```python
from build123d import *

# Parameters (mm, degrees)
CROQUIS1_W                 = 35
CROQUIS1_H                 = 35
CROQUIS1_R                 = 1.25
SALIENTE_EXTRUIR1_DEPTH    = 5
SALIENTE_EXTRUIR2_DEPTH    = 35
CORTAR_EXTRUIR2_DEPTH      = 41.51542916
CORTAR_EXTRUIR2_DEPTH_BACK = 41.51542916
CROQUIS4_R                 = 1.25
CORTAR_EXTRUIR3_DEPTH      = 10
CROQUIS5_R                 = 3
CORTAR_EXTRUIR6_DEPTH      = 4.1


with BuildPart() as part:
    # Croquis1 → Saliente-Extruir1 (new body)
    with BuildSketch(Plane.XY):
        Rectangle(CROQUIS1_W, CROQUIS1_H)
        with Locations((15.37, -15.37)):
            Circle(CROQUIS1_R, mode=Mode.SUBTRACT)
        with Locations((-15.37, -15.37)):
            Circle(CROQUIS1_R, mode=Mode.SUBTRACT)
        with Locations((-15.37, 15.37)):
            Circle(CROQUIS1_R, mode=Mode.SUBTRACT)
        with Locations((15.37, 15.37)):
            Circle(CROQUIS1_R, mode=Mode.SUBTRACT)
    extrude(amount=SALIENTE_EXTRUIR1_DEPTH)

    # Croquis2 → Saliente-Extruir2 (add, through all)
    with BuildSketch(Plane(origin=(0, 17.5, 0), x_dir=(1, 0, 0), z_dir=(0, 1, 0))):
        with BuildLine():
            Line((17.5, -5), (17.5, -10.5))
            ThreePointArc((17.5, -10.5), (13.206356105, -6.465716172), (7.5, -5))
            Line((7.5, -5), (17.5, -5))
        make_face()
    extrude(amount=-SALIENTE_EXTRUIR2_DEPTH)

    # Croquis3 → Cortar-Extruir2 (cut, two sides: drawn at the far end of the back side and taken through both)
    with BuildSketch(Plane(origin=(0, 17.5, 0), x_dir=(1, 0, 0), z_dir=(0, 1, 0)).offset(-CORTAR_EXTRUIR2_DEPTH_BACK)):
        with BuildLine():
            Line((17.5, 0), (7.5, 0))
            ThreePointArc((7.5, 0), (13.147178499, -1.392279049), (17.5, -5.25))
            Line((17.5, -5.25), (17.5, 0))
        make_face()
    extrude(amount=CORTAR_EXTRUIR2_DEPTH + CORTAR_EXTRUIR2_DEPTH_BACK, mode=Mode.SUBTRACT)

    # Croquis4 → Cortar-Extruir3 (cut)
    with BuildSketch(Plane(origin=(0, 0, 5), x_dir=(-1, 0, 0), z_dir=(0, 0, -1))):
        with Locations((-15.37, 15.37)):
            Circle(CROQUIS4_R)
        with Locations((-15.37, -15.37)):
            Circle(CROQUIS4_R)
    extrude(amount=-CORTAR_EXTRUIR3_DEPTH, mode=Mode.SUBTRACT)

    # Croquis5 → Cortar-Extruir6 (cut)
    with BuildSketch(Plane(origin=(0, 0, 0), x_dir=(-1, 0, 0), z_dir=(0, 0, -1))):
        with Locations((-15.37, 15.37)):
            Circle(CROQUIS5_R)
        with Locations((-15.37, -15.37)):
            Circle(CROQUIS5_R)
    extrude(amount=-CORTAR_EXTRUIR6_DEPTH, mode=Mode.SUBTRACT)


solid = part.part
```
Can you work these out from the model? Positions are in its coordinate system, mm. Give positions to 0.01 mm unless a question says otherwise; leave off trailing zeros. Write each loop counter-clockwise with the first axis right and the second up, starting at its lowest first coordinate (ties: lowest second). Pieces come first, ordered by that corner, then holes. Notation, with made-up numbers: (-18, 21) -> (-7, 21) arc R29 ccw to (-7, 49) -> close; hole circle Ø1 at (41.5, 25). An arc over 180 degrees is marked (long way). One line per item, written item: value.
Q1. We'd pull the mould along X, two halves only. Please class faces 1 (the face through (-14.18, 15.75, 2.46)), 2 (the face through (-17.5, 0, 2)), 3 (the face through (-5, 0, 5)), 4 (the face through (13.07, -0.24, 1.35)): +X half, -X half, draft (parallel to the pull), parting line (faces both ways), or undercut.
Results found:
face 1: undercut
face 2: -X half
face 3: draft
face 4: +X half
Q2. For P1, Ø12, axis at x = -8, y = -7, coming from the +Z side; P2, Ø2, axis at x = 15.5, y = 14, coming from the -Z side; P3, Ø3, axis at x = 15.37, y = -15.37, coming from the +Z side, each with a flat end and sliding along its axis, tell me the tip position at first contact or that it passes through.
Results found:
P1: stops at z = 5
P2: stops at z = 4.1
P3: stops at z = 9.6
Q3. Please list where these lines run through material, in increasing order: line 1 (Y direction, x = 15.37, z = 4.8); line 2 (Z direction, x = -9, y = -14); line 3 (X direction, y = -15.37, z = 8.35). Write a range as [from, to].
Results found:
line 1: y = [-17.5, -16.62], [-14.12, 14.12], [16.62, 17.5]
line 2: z = [0, 5]
line 3: x = [16.62, 17.5]
Q4. Imagine slicing it at A-A on x = -15.37. Please give me the cut outline in (y, z).
Results found:
outline: (-17.5, 0) -> (-16.62, 0) -> (-16.62, 5) -> (-17.5, 5) -> close; (-14.12, 0) -> (14.12, 0) -> (14.12, 5) -> (-14.12, 5) -> close; (16.62, 0) -> (17.5, 0) -> (17.5, 5) -> (16.62, 5) -> close
Q5. Imagine slicing it at B-B on z = 3.5. Please give me the cut outline in (x, y).
Results found:
outline: (-17.5, -17.5) -> (13.26, -17.5) arc R3 cw to (16.03, -12.44) -> (16.03, 12.44) arc R3 cw to (13.26, 17.5) -> (-17.5, 17.5) -> close; hole circle Ø2.5 at (-15.37, -15.37); hole circle Ø2.5 at (-15.37, 15.37)
Q6. Imagine slicing it at C-C on y = 5.5. Please give me the cut outline in (x, z), and give its area (3 significant figures).
Results found:
outline: (-17.5, 0) -> (7.5, 0) arc R12.15 ccw to (17.5, 5.25) -> (17.5, 10.5) arc R11.84 cw to (7.5, 5) -> (-17.5, 5) -> close
area: 176 mm^2
Q7. Imagine slicing it at D-D on z = 8.75. Please give me the cut outline in (x, y), and give its area (3 significant figures).
Results found:
outline: (16.15, -17.5) -> (17.5, -17.5) -> (17.5, 17.5) -> (16.15, 17.5) -> (16.15, 16.35) arc R1.25 cw to (16.15, 14.39) -> (16.15, -14.39) arc R1.25 cw to (16.15, -16.35) -> close
area: 46.1 mm^2
